from build123d import *

# Parameters (mm, degrees)
F0_R     = 73.2052384523
F1_DEPTH = 2.54
F0_W     = 152.1742939949
F0_H     = 151.6839265823
F2_DEPTH = 25.4
F4_DEPTH = 25.4


with BuildPart() as f1:
    # F0 (on Top) → F1 (new body)
    with BuildSketch(Plane.XY):
        Circle(F0_R)
        Polygon((-40.7538563013, -37.2341535985), (-63.2713064551, -18.5253843665), (-28.52431871, 54.2785041034), (0, 22.3221629858), (28.1545463949, 54.3052591383), (63.3123517036, -18.7383014709), (40.8359244466, -37.5453457236), (21.7867922038, 16.0413701087), (0, -9.6461987123), (-22.1097543836, 15.8388335258), align=None, mode=Mode.SUBTRACT)
    extrude(amount=F1_DEPTH)

    # F0 (on Top) → F2 (join)
    with BuildSketch(Plane.XY):
        Rectangle(F0_W, F0_H)
        Circle(F0_R, mode=Mode.SUBTRACT)
    extrude(amount=F2_DEPTH)

    # F3 (on face) → F4 (join)
    with BuildSketch(Plane.XY.offset(25.4)):
        Polygon((-28.52431871, 54.2785041034), (-63.2713064551, -18.5253843665), (-40.7538563013, -37.2341535985), (-22.1097543836, 15.8388335258), (0, -9.6461987123), (21.7867922038, 16.0413701087), (40.8359244466, -37.5453457236), (63.3123517036, -18.7383014709), (28.1545463949, 54.3052591383), (0, 22.3221629858), align=None)
    extrude(amount=-F4_DEPTH)


solid = f1.part
Source: CAD feature listing. Evaluate the final solid. Frame: model axes, mm. A direction names the side the tool comes from. Give positions to 0.01 mm unless a question says otherwise; leave off trailing zeros. Write each loop counter-clockwise with the first axis right and the second up, starting at its lowest first coordinate (ties: lowest second). Pieces come first, ordered by that corner, then holes. Notation, with made-up numbers: M 30.25,-28 L 78.25,-28 A19 cw 78.25,7 Z; hole C 89,20 d4. An arc over 180 degrees is marked long. Return JSON: item names as keys, results as strings. Group by question number.
1) Set-up query: faces 4 (the face through (-15.869, -71.464, 13.81)), 5 (the face through (-62.4, -39, 25.4)). Return all of +Z, -Z, +X, -X, +Y, -Y with unobstructed straight access to the full face (end or side cutting, diameter ignored); none if empty.
2) Material intervals for line 1 along Y through (x, z) = (0, 15.25); line 2 along Y through (x, z) = (17, 11.75); line 3 along X through (y, z) = (-25, 6), sorted ascending. Write a range as [from, to].
3) Cut plane A-A, the plane z = 10.75. Output: boundary loops of the cut face in (x, y).
4) Cut plane C-C, the plane y = 34.5. Output: boundary loops of the cut face in (x, z), plus the area to 3 significant figures.
5) Pull-direction query (Y, two-part tool) for faces 1 (the face through (76.087, -1, 13)), 2 (the face through (-1, -75.842, 13)), 3 (the face through (-31.562, -11.069, 14.13)); classes: pulls with the +Y half, pulls with the -Y half, needs draft (parallel to the pull), parting line crosses it, or undercut.
6) Cut plane D-D, the plane x = 15. Output: boundary loops of the cut face in (y, z), plus the area to 3 significant figures.
7) Pin query (flat end, axial travel): P1, Ø1, axis at x = -20, y = 10.5, coming from the -Z side; P2, Ø4, axis at x = -46.5, y = 49.5, coming from the +Z side. Return the tip coordinate at first contact, or that it passes through.
8) Cut plane B-B, the plane x = 61. Output: boundary loops of the cut face in (y, z).
Recorded:
{
 "1": {"face 4": "+Z", "face 5": "+Z, +X, -X, +Y, -Y"},
 "2": {"line 1": "y = [-75.84, -73.21], [-9.65, 22.32], [73.21, 75.84]", "line 2": "y = [-75.84, -71.2], [10.4, 41.63], [71.2, 75.84]", "line 3": "x = [-76.09, -68.8], [-55.48, -36.46], [36.38, 55.83], [68.8, 76.09]"},
 "3": {"outline": "M -76.09,-75.84 L 76.09,-75.84 L 76.09,75.84 L -76.09,75.84 Z; M -63.27,-18.53 L -40.75,-37.23 L -22.11,15.84 L 0,-9.65 L 21.79,16.04 L 40.84,-37.55 L 63.31,-18.74 L 28.15,54.31 L 0,22.32 L -28.52,54.28 Z; hole C 0,0 d146.41"},
 "4": {"outline": "M -76.09,0 L 76.09,0 L 76.09,25.4 L 64.57,25.4 L 64.57,2.54 L 37.69,2.54 L 37.69,25.4 L 10.72,25.4 L 10.72,2.54 L -10.87,2.54 L -10.87,25.4 L -37.96,25.4 L -37.96,2.54 L -64.57,2.54 L -64.57,25.4 L -76.09,25.4 Z", "area": "2,150 mm²"},
 "5": {"face 1": "needs draft", "face 2": "pulls with the -Y half", "face 3": "undercut"},
 "6": {"outline": "M -75.84,0 L 75.84,0 L 75.84,25.4 L 71.65,25.4 L 71.65,2.54 L 39.36,2.54 L 39.36,25.4 L 8.04,25.4 L 8.04,2.54 L -71.65,2.54 L -71.65,25.4 L -75.84,25.4 Z", "area": "1,290 mm²"},
 "7": {"P1": "stops at z = 0", "P2": "stops at z = 2.54"},
 "8": {"outline": "M -75.84,0 L 75.84,0 L 75.84,25.4 L 40.47,25.4 L 40.47,2.54 L -13.93,2.54 L -13.93,25.4 L -20.67,25.4 L -20.67,2.54 L -40.47,2.54 L -40.47,25.4 L -75.84,25.4 Z"}
}
